from build123d import *

# Parameters (mm, degrees)
SKETCH2_W           = 60
SKETCH2_H           = 28
BOSS_EXTRUDE1_DEPTH = 3
SKETCH3_R           = 2
CUT_EXTRUDE1_DEPTH  = 4


with BuildPart() as part:
    # Sketch2 → Boss-Extrude1 (new body)
    with BuildSketch(Plane(origin=(0, 0, 0), x_dir=(1, 0, 0), z_dir=(0, 1, 0))):
        with Locations((30, 14)):
            Rectangle(SKETCH2_W, SKETCH2_H)
    extrude(amount=BOSS_EXTRUDE1_DEPTH)

    # Sketch3 → Cut-Extrude1 (cut, through all)
    with BuildSketch(Plane(origin=(0, 3, 0), x_dir=(1, 0, 0), z_dir=(0, 1, 0))):
        with Locations((4, 4)):
            Circle(SKETCH3_R)
        with Locations((4, 24)):
            Circle(SKETCH3_R)
        with Locations((56, 24)):
            Circle(SKETCH3_R)
        with Locations((56, 4)):
            Circle(SKETCH3_R)
    extrude(amount=-CUT_EXTRUDE1_DEPTH, mode=Mode.SUBTRACT)


solid = part.part
Can you work these out from the model? Positions are in its coordinate system, mm. Coordinates: 2 decimals unless noted, no trailing zeros. Loops run counter-clockwise (first coordinate to the right, second up) from the corner with the lowest first, then second, coordinate; pieces in that order, holes last. Notation, with made-up numbers: (59, 59) - (111, 59) arc R31 cw to (111, 97) - close; hole circle Ø10 at (-20.75, 35.25). An arc over 180 degrees is marked (long way). Put each result on its own line as item: value. Start each with the question number.
Item 1: For pin 1 (3.5 mm diameter, centred on x = 4, z = -4, fed in from +Y); pin 2 (6.5 mm diameter, centred on x = 4, z = -24, fed in from -Y), each with a flat end and sliding along its axis, tell me the tip position at first contact or that it passes through.
Item 2: Suppose I cut it at A-A (x = 4). Please give me the cut outline in (y, z), and give its area (3 significant figures).
Item 3: If I drill on line 1 along Z through (x, y) = (4, 2.2); line 2 along X through (y, z) = (1.3, -4), over which ranges is the centre line in solid material (lowest first)?
Item 4: Suppose I cut it at C-C (y = 0.95). Please give me the cut outline in (x, z), and give its area (3 significant figures).
Item 5: Suppose I cut it at B-B (z = -4). Please give me the cut outline in (x, y).
Item 6: If we mould it in two halves opening along Z, with no side actions, what happens to faces 1 (the face through (0, 1, -14)), 2 (the face through (54.4, 1.5, -22.8)), 3 (the face through (2.4, 1.5, -2.8)), 4 (the face through (30, 1, -28))? For each: +Z half, -Z half, draft (parallel to the pull), parting line (faces both ways), or undercut.
Here are the results:
1. pin 1: through
1. pin 2: y = 0
2. outline: (0, -28) - (3, -28) - (3, -26) - (0, -26) - close; (0, -22) - (3, -22) - (3, -6) - (0, -6) - close; (0, -2) - (3, -2) - (3, 0) - (0, 0) - close
2. area: 60.0 mm²
3. line 1: -28 to -26, -22 to -6, -2 to 0
3. line 2: 0 to 2, 6 to 54, 58 to 60
4. outline: (0, -28) - (60, -28) - (60, 0) - (0, 0) - close; hole circle Ø4 at (4, -24); hole circle Ø4 at (4, -4); hole circle Ø4 at (56, -24); hole circle Ø4 at (56, -4)
4. area: 1,630 mm²
5. outline: (0, 0) - (2, 0) - (2, 3) - (0, 3) - close; (6, 0) - (54, 0) - (54, 3) - (6, 3) - close; (58, 0) - (60, 0) - (60, 3) - (58, 3) - close
6. face 1: draft
6. face 2: undercut
6. face 3: undercut
6. face 4: -Z half
